Here's how the part is built. I have some questions about the finished solid (model axes, mm). A direction names the side the tool comes from. Round coordinates to 2 decimals unless told otherwise and drop trailing zeros. Write each loop counter-clockwise with the first axis right and the second up, starting at its lowest first coordinate (ties: lowest second). Pieces come first, ordered by that corner, then holes. Notation, with made-up numbers: M -32.75,-23 L 7.25,-23 A12 cw 7.25,-19 Z; hole C 17.5,49 d2. An arc over 180 degrees is marked long. Write item = value, one per line. Start each with the question number.
(1) I want a section at B-B (y = 63.5). List the corners of the cut face in (x, z) for me, and give its area (3 significant figures).
(2) I want a section at C-C (z = -6). List the corners of the cut face in (x, y) for me, and give its area (3 significant figures).
(3) I need wall thicknesses on line 1 along Z through (x, y) = (-27.5, 47.5); line 2 along Y through (x, z) = (-21, -5.5); line 3 along Y through (x, z) = (21, 17.5). Which ranges of each line are inside material? Lowest first, please.
(4) If we mould it in two halves opening along Z, with no side actions, what happens to faces 1 (the flat face through (-19, 39, -11.928)), 2 (the cylindrical face through (-23.25, 58.58, 23.14)), 3 (the flat face through (-20, 5, -36.928)), 4 (the flat face through (-19, 17.5, 3))? For each: released by +Z, released by -Z, zero draft, split by the parting line, or undercut.
(5) On a 3-axis mill with a long thin cutter (end or side, diameter ignored), from which of +Z, -Z, +X, -X, +Y, -Y can I reach the whole of each face in a straight line? I mean faces 5 (the flat face through (-20, 35, 28.072)), 6 (the flat face through (-20, 35, -21.928)), 7 (the flat face through (-19, 40, 18.072)). Say none if no direction works.
(6) I want a section at D-D (z = -17). List the corners of the cut face in (x, y) for me, and give its area (3 significant figures).
(7) I want a section at A-A (y = 22). List the corners of the cut face in (x, z) for me, and give its area (3 significant figures).
(8) Will these pins go through, and if not, where does the flat tip stop? pin 1 Ø17 at (x, y) = (-5, 45) entering from -Z; pin 2 Ø6 at (x, y) = (-19.28, 61.62) entering from -Z; pin 3 Ø9 at (x, z) = (-18.5, -1) entering from +Y; pin 4 Ø5 at (x, z) = (-12.5, -23.5) entering from +Y.
```python
from build123d import *

# Parameters (mm, degrees)
SKETCH1_W           = 100
SKETCH1_H           = 80
BOSS_EXTRUDE1_DEPTH = 10
SKETCH2_W           = 70
SKETCH2_H           = 50
BOSS_EXTRUDE2_DEPTH = 65
CUT_EXTRUDE2_DEPTH  = 94
SKETCH3_R           = 5
CUT_EXTRUDE4_DEPTH  = 94


with BuildPart() as part:
    # Sketch1 → Boss-Extrude1 (new body)
    with BuildSketch(Plane(origin=(0, 0, 0), x_dir=(1, 0, 0), z_dir=(0, 1, 0))):
        with Locations((-19.281045752, -3.071895425)):
            Rectangle(SKETCH1_W, SKETCH1_H)
    extrude(amount=BOSS_EXTRUDE1_DEPTH)

    # Sketch2 → Boss-Extrude2 (add)
    with BuildSketch(Plane(origin=(0, 10, 0), x_dir=(1, 0, 0), z_dir=(0, 1, 0))):
        with Locations((-19.281045752, -3.071895425)):
            Rectangle(SKETCH2_W, SKETCH2_H)
    extrude(amount=BOSS_EXTRUDE2_DEPTH)

    # Sketch5 → Cut-Extrude2 (cut)
    with BuildSketch(Plane(origin=(15.718954248, 0, 0), x_dir=(0, 0, -1), z_dir=(1, 0, 0))):
        Polygon((11.928104575, 17.5), (-18.071895425, 17.5), (-18.071895425, 67.5), (-18.071895425, 75), (11.928104575, 75), (11.928104575, 67.5), align=None)
    extrude(amount=-CUT_EXTRUDE2_DEPTH, mode=Mode.SUBTRACT)

    # Sketch3 → Cut-Extrude4 (cut)
    with BuildSketch(Plane.XY.offset(28.071895425)):
        Polygon((-54.281045752, 75), (-54.281045752, 10), (-31.2976006, 67.501159063), (-28.300283638, 75), align=None)
        with BuildLine():
            Line((-28.300283638, 75), (-31.2976006, 67.501159063))
            ThreePointArc((-31.2976006, 67.501159063), (-26.363245371, 72.97149148), (-19.281045752, 75))
            Line((-19.281045752, 75), (-28.300283638, 75))
        make_face()
        with BuildLine():
            Line((-10.261807865, 75), (-19.281045752, 75))
            ThreePointArc((-19.281045752, 75), (-12.198846132, 72.97149148), (-7.264490904, 67.501159063))
            Line((-7.264490904, 67.501159063), (-10.261807865, 75))
        make_face()
        Polygon((-10.261807865, 75), (-7.264490904, 67.501159063), (15.718954248, 10), (15.718954248, 75), align=None)
        with Locations((-19.281045752, 61.622585577)):
            Circle(SKETCH3_R)
    extrude(amount=-CUT_EXTRUDE4_DEPTH, mode=Mode.SUBTRACT)


solid = part.part
```
Returned:
q1.outline = M -32.9,-21.93 L -23.92,-21.93 L -23.92,-11.93 L -32.9,-11.93 Z; M -32.9,18.07 L -23.92,18.07 L -23.92,28.07 L -32.9,28.07 Z; M -14.65,-21.93 L -5.67,-21.93 L -5.67,-11.93 L -14.65,-11.93 Z; M -14.65,18.07 L -5.67,18.07 L -5.67,28.07 L -14.65,28.07 Z
q1.area = 359 mm²
q2.outline = M -69.28,0 L 30.72,0 L 30.72,10 L 15.72,10 L 12.72,17.5 L -51.28,17.5 L -54.28,10 L -69.28,10 Z
q2.area = 1,500 mm²
q3.line_1 = -21.93 to -11.93, 18.07 to 28.07
q3.line_2 = 0 to 17.5
q3.line_3 = 0 to 10
q4.face_1 = undercut
q4.face_2 = zero draft
q4.face_3 = released by -Z
q4.face_4 = undercut
q5.face_5 = +Z, +X, -X, +Y
q5.face_6 = -Z, +X, -X, +Y
q5.face_7 = +X, -X, +Y
q6.outline = M -69.28,0 L 30.72,0 L 30.72,10 L 15.72,10 L -7.26,67.5 A13.38 ccw -31.3,67.5 L -54.28,10 L -69.28,10 Z; hole C -19.28,61.62 d10
q6.area = 3,750 mm²
q7.outline = M -49.48,-21.93 L 10.92,-21.93 L 10.92,-11.93 L -49.48,-11.93 Z; M -49.48,18.07 L 10.92,18.07 L 10.92,28.07 L -49.48,28.07 Z
q7.area = 1,210 mm²
q8.pin_1 = -21.93
q8.pin_2 = through
q8.pin_3 = 17.5
q8.pin_4 = 74.09
